from build123d import *

# Parameters (mm, degrees)
CROQUIS1_W              = 60
CROQUIS1_H              = 60
SALIENTE_EXTRUIR1_DEPTH = 3


with BuildPart() as part:
    # Croquis1 → Saliente-Extruir1 (new body)
    with BuildSketch(Plane(origin=(0, 0, 0), x_dir=(1, 0, 0), z_dir=(0, 1, 0))):
        Rectangle(CROQUIS1_W, CROQUIS1_H)
        Polygon((0, 10), (-4, 10), (-4, 7), (4, 7), (4, 10), align=None, mode=Mode.SUBTRACT)
        Polygon((7, 4), (7, -4), (10, -4), (10, 0), (10, 4), align=None, mode=Mode.SUBTRACT)
        Polygon((4, -7), (-4, -7), (-4, -10), (0, -10), (4, -10), align=None, mode=Mode.SUBTRACT)
        Polygon((-7, -4), (-7, 4), (-10, 4), (-10, 0), (-10, -4), align=None, mode=Mode.SUBTRACT)
        Polygon((20, 1.5), (16, 1.5), (16, -1.5), (24, -1.5), (24, 1.5), align=None, mode=Mode.SUBTRACT)
        Polygon((1.5, -20), (1.5, -16), (-1.5, -16), (-1.5, -24), (1.5, -24), align=None, mode=Mode.SUBTRACT)
        Polygon((-20, -1.5), (-16, -1.5), (-16, 1.5), (-24, 1.5), (-24, -1.5), align=None, mode=Mode.SUBTRACT)
        Polygon((-1.5, 20), (-1.5, 16), (1.5, 16), (1.5, 24), (-1.5, 24), align=None, mode=Mode.SUBTRACT)
    extrude(amount=SALIENTE_EXTRUIR1_DEPTH)


solid = part.part
Can you work these out from the model? Positions are in its coordinate system, mm. A direction names the side the tool comes from. Coordinates: 2 decimals unless noted, no trailing zeros. Loops run counter-clockwise (first coordinate to the right, second up) from the corner with the lowest first, then second, coordinate; pieces in that order, holes last. Notation, with made-up numbers: (74.25, 77.5) - (118.25, 77.5) arc R7 cw to (118.25, 84.5) - close; hole circle Ø2 at (42.25, 30.5). An arc over 180 degrees is marked (long way). Answer as a JSON object with one key per item and string values. Group by question number.
Item 1: If we section it at A-A (z = -21): List the corners of the cut face in (x, y) for me, plus the area to 3 significant figures.
Item 2: For pin 1 (5 mm diameter, centred on x = 11, z = 1.5, fed in from -Y), with a flat end and sliding along its axis, tell me the tip position at first contact or that it passes through.
Item 3: If I drill on L1, parallel to Z at x = 3, y = 2.1; L2, parallel to Z at x = 23, y = 2.65, over which ranges is the centre line in solid material (lowest first)? Write a range as from..to.
Item 4: If we mould it in two halves opening along Z, with no side actions, what happens to faces 1 (the face through (0, 1, 16)), 2 (the face through (0, 1, 30)), 3 (the face through (0, 0, 0))? For each: released by +Z, released by -Z, zero draft, split by the parting line, or undercut.
Item 5: If we section it at C-C (z = 2.5): List the corners of the cut face in (x, y) for me.
Item 6: If we section it at D-D (x = 9): List the corners of the cut face in (y, z) for me.
Item 7: On a 3-axis mill with a long thin cutter (end or side, diameter ignored), from which of +Z, -Z, +X, -X, +Y, -Y can I reach the whole of each face in a straight line? I mean faces 4 (the face through (-4, 1, 8)), 5 (the face through (-30, 1, 0)). Say none if no direction works.
Returned:
{
 "1": {"outline": "(-30, 0) - (-1.5, 0) - (-1.5, 3) - (-30, 3) - close; (1.5, 0) - (30, 0) - (30, 3) - (1.5, 3) - close", "area": "171 mm²"},
 "2": {"pin 1": "stops at y = 0"},
 "3": {"L1": "z = -30..-10, -7..7, 10..30", "L2": "z = -30..-1.5, 1.5..30"},
 "4": {"face 1": "undercut", "face 2": "released by +Z", "face 3": "zero draft"},
 "5": {"outline": "(-30, 0) - (-10, 0) - (-10, 3) - (-30, 3) - close; (-7, 0) - (7, 0) - (7, 3) - (-7, 3) - close; (10, 0) - (30, 0) - (30, 3) - (10, 3) - close"},
 "6": {"outline": "(0, -30) - (3, -30) - (3, -4) - (0, -4) - close; (0, 4) - (3, 4) - (3, 30) - (0, 30) - close"},
 "7": {"face 4": "+Y, -Y", "face 5": "+Z, -Z, -X, +Y, -Y"}
}
